```python
from build123d import *

# Parameters (mm, degrees)
F1_DEPTH = 3.81
F2_R     = 3.81
F3_DEPTH = 4.064
F5_D     = 2.54
F5_DEPTH = 12.7


with BuildPart() as f1:
    # F0 (on Top) → F1 (new body)
    with BuildSketch(Plane.XY):
        with BuildLine():
            Line((0, 93.98), (0, 5.08))
            ThreePointArc((0, 5.08), (5.08, 0), (10.16, 5.08))
            Line((10.16, 5.08), (10.16, 93.98))
            ThreePointArc((10.16, 93.98), (5.08, 99.06), (0, 93.98))
        make_face()
    extrude(amount=F1_DEPTH)

    # F2 (on face) → F3 (join)
    with BuildSketch(Plane.XY.offset(3.81)):
        with Locations((5.08, 5.08)):
            Circle(F2_R)
    extrude(amount=F3_DEPTH)

    # F5
    with Locations(Plane.XY.offset(7.874)):
        with Locations((5.08, 5.08)):
            Hole(F5_D / 2, depth=F5_DEPTH)


solid = f1.part
```
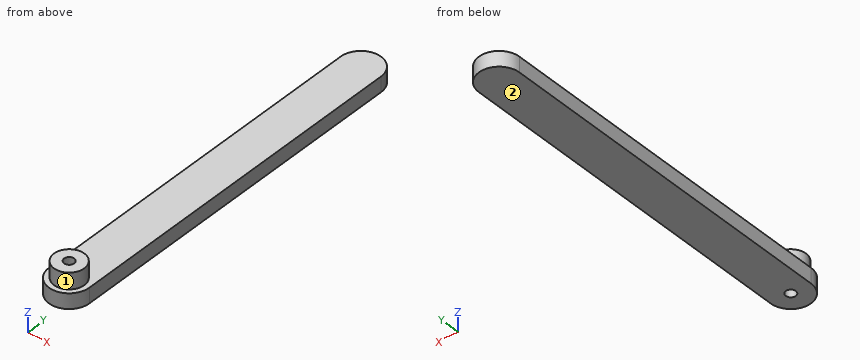
CAD build for the part. Positions are in the model's coordinates, mm. Face numbers are marked on the shaded views. A direction names the side the tool comes from. Coordinates: 2 decimals unless noted, no trailing zeros. Write each loop counter-clockwise with the first axis right and the second up, starting at its lowest first coordinate (ties: lowest second). Pieces come first, ordered by that corner, then holes.
(1) Cut at B-B, the plane y = 66. List the corners of the cut face in (x, z), and give its area (3 significant figures).
(2) Flat gauge pin, fed straight in: pin 1 (2 mm diameter, centred on x = 1.5, y = 44, fed in from +Z). Where does the tip first touch, or does it go through?
(3) 3-axis set-ups, long thin cutter, end or side, ignore diameter. For the marked faces 1 and 2: which of +Z, -Z, +X, -X, +Y, -Y reach the whole face in a straight line?
(4) Cut at A-A, the plane x = 5.08. List the corners of the cut face in (y, z).
(5) Drill centre lines: probe 1 along Y at (x, z) = (5.08, 5); probe 2 along Y at (x, z) = (5.08, 2.75); probe 3 along Z at (x, y) = (2.5, 18.5). Where is each one in solid material? Low to high.
Geometry says:
1. outline: (0, 0) - (10.16, 0) - (10.16, 3.81) - (0, 3.81) - close
1. area: 38.7 mm2
2. pin 1: stops at z = 3.81
3. face 1: +Z
3. face 2: -Z, +X, -X, +Y, -Y
4. outline: (0, 0) - (3.81, 0) - (3.81, 7.87) - (1.27, 7.87) - (1.27, 3.81) - (0, 3.81) - close; (6.35, 0) - (99.06, 0) - (99.06, 3.81) - (8.89, 3.81) - (8.89, 7.87) - (6.35, 7.87) - close
5. probe 1: y = 1.27 to 3.81, 6.35 to 8.89
5. probe 2: y = 0 to 3.81, 6.35 to 99.06
5. probe 3: z = 0 to 3.81
